```python
from build123d import *

# Parameters (mm, degrees)
SKETCH_1_W          = 12
SKETCH_1_H          = 12
SKETCH_1_W_2        = 10
SKETCH_1_H_2        = 10
EXTRUDE_1_DEPTH     = 410
SKETCH_2_R          = 1.35
CUT_EXTRUDE_1_DEPTH = 411.219453464
SKETCH_3_R          = 1.35
CUT_EXTRUDE_2_DEPTH = 411.219453464
SKETCH_4_R          = 1.35
CUT_EXTRUDE_3_DEPTH = 411.219453464


with BuildPart() as part:
    # 草图1 → 凸台-拉伸1 (new body)
    with BuildSketch(Plane(origin=(0, 0, 0), x_dir=(1, 0, 0), z_dir=(0, 1, 0))):
        Rectangle(SKETCH_1_W, SKETCH_1_H)
        Rectangle(SKETCH_1_W_2, SKETCH_1_H_2, mode=Mode.SUBTRACT)
    extrude(amount=EXTRUDE_1_DEPTH)

    # 草图2 → 切除-拉伸1 (cut, through all)
    with BuildSketch(Plane(origin=(6, 0, 0), x_dir=(0, 0, -1), z_dir=(1, 0, 0))):
        with Locations((0, 5)):
            Circle(SKETCH_2_R)
        with Locations((0, 17)):
            Circle(SKETCH_2_R)
        with Locations((0, 51)):
            Circle(SKETCH_2_R)
    extrude(amount=-CUT_EXTRUDE_1_DEPTH, mode=Mode.SUBTRACT)

    # 草图3 → 切除-拉伸2 (cut, through all)
    with BuildSketch(Plane(origin=(6, 0, 0), x_dir=(0, 0, -1), z_dir=(1, 0, 0))):
        with Locations((0, 407)):
            Circle(SKETCH_3_R)
        with Locations((0, 397)):
            Circle(SKETCH_3_R)
    extrude(amount=-CUT_EXTRUDE_2_DEPTH, mode=Mode.SUBTRACT)

    # 草图4 → 切除-拉伸3 (cut, through all)
    with BuildSketch(Plane(origin=(0, 0, -6), x_dir=(-1, 0, 0), z_dir=(0, 0, -1))):
        with Locations((0, 45)):
            Circle(SKETCH_4_R)
        with Locations((0, 57)):
            Circle(SKETCH_4_R)
    extrude(amount=-CUT_EXTRUDE_3_DEPTH, mode=Mode.SUBTRACT)


solid = part.part
```
Verification items for the finished model (mm, model axes). A direction names the side the tool comes from. Round coordinates to 2 decimals unless told otherwise and drop trailing zeros. Write each loop counter-clockwise with the first axis right and the second up, starting at its lowest first coordinate (ties: lowest second). Pieces come first, ordered by that corner, then holes. Notation, with made-up numbers: (78, -25.75) - (87, -25.75) arc R23 ccw to (87, -5.75) - close; hole circle Ø5 at (-23, 60.25). An arc over 180 degrees is marked (long way). Answer as a JSON object with one key per item and string values. Group by question number.
Q1. Mould release check, pull along Z, two halves, no side actions. Record for faces 3 (the flat face through (-6, 202, 0)), 4 (the flat face through (0, 202, 6)), 5 (the flat face through (-5, 202, 0)): released by +Z, released by -Z, zero draft, split by the parting line, or undercut.
Q2. Tool access check on faces 1 (the flat face through (5, 202, 0)), 2 (the flat face through (6, 202, 0)). Record the directions out of +Z, -Z, +X, -X, +Y, -Y that give a thin tool (end or side, any length) a straight path to the whole face; none if there is none.
Q3. Section check A-A, the plane y = 250.5. Enter the section's corners in (x, z).
Q4. Thickness scan on line 1 (Y direction, x = 0, z = -5.45); line 2 (Y direction, x = 5.25, z = 0); line 3 (Z direction, x = 3.25, y = 329). Record the ranges inside material, lowest first.
Found:
{
 "1": {"face 3": "zero draft", "face 4": "released by +Z", "face 5": "undercut"},
 "2": {"face 1": "+Y, -Y", "face 2": "+Z, -Z, +X, +Y, -Y"},
 "3": {"outline": "(-6, -6) - (6, -6) - (6, 6) - (-6, 6) - close; hole (-5, -5) - (5, -5) - (5, 5) - (-5, 5) - close"},
 "4": {"line 1": "y = 0 to 43.65, 46.35 to 55.65, 58.35 to 410", "line 2": "y = 0 to 3.65, 6.35 to 15.65, 18.35 to 49.65, 52.35 to 395.65, 398.35 to 405.65, 408.35 to 410", "line 3": "z = -6 to -5, 5 to 6"}
}
